Input: part model. Units: mm. Frame: model coordinates. A direction names the side the tool comes from. Round coordinates to 2 decimals unless told otherwise and drop trailing zeros. Order: outer loops, then holes, each group sorted by start corner. A loop starts at its lowest first (then second) coordinate and runs counter-clockwise, first axis right, second up.
Item 1: Cut plane B-B on z = 20.5. Output: boundary loops of the cut face in (x, y).
Item 2: Cut plane D-D on y = -0.8. Give the number of separate pieces and of enclosed holes in the cut face, then the cut area to 3 significant figures.
Item 3: Reachability of faces 1 (the cylindrical face through (23.359, -1.479, -10.926)), 2 (the cylindrical face through (79.533, -1.479, -7.956)), 3 (the cylindrical face through (79.588, -1.479, 7.981)) from +Z, -Z, +X, -X, +Y, -Y: full face, straight path, thin tool, end or side. Return the list, or none.
Item 4: Cut plane A-A on x = 105. Output: boundary loops of the cut face in (y, z).
Item 5: Line query: L1, parallel to X at y = -1.85, z = 22; L2, parallel to X at y = -0.3, z = -17; L3, parallel to X at y = -0.55, z = 5. Output: solid intervals per line, ascending.
Item 6: Cut plane C-C on z = 4. Output: boundary loops of the cut face in (x, y), then the cut area to 3 significant figures.
Item 7: First-contact query: pin 1 (12 mm diameter, centred on x = 19.5, z = 5.5, fed in from +Y); pin 2 (1.5 mm diameter, centred on x = 38, y = -1.5, fed in from -Z); pin 3 (0.9 mm diameter, centred on x = 65, y = -1.5, fed in from +Z); pin 4 (8 mm diameter, centred on x = 105, z = -22, fed in from -Y). Flat tips, straight axial feed; report the tip coordinate or a pass-through.
```python
from build123d import *

# Parameters (mm, degrees)
BASE_DEPTH    = 3
SKETCH2_R     = 6.5
HOLES_DEPTH   = 120.406867474
CUTAWAY_DEPTH = 120.406867474


with BuildPart() as part:
    # Sketch1 → base (new body)
    with BuildSketch(Plane(origin=(0, 0, 0), x_dir=(1, 0, 0), z_dir=(0, 1, 0))):
        with BuildLine():
            Line((-10, -22), (-10, 22))
            ThreePointArc((-10, 22), (-7.071067812, 29.071067812), (0, 32))
            Line((0, 32), (17, 32))
            ThreePointArc((17, 32), (21.226182617, 31.06307787), (24.660444431, 28.427876097))
            Line((24.660444431, 28.427876097), (40.722333621, 9.286061952))
            ThreePointArc((40.722333621, 9.286061952), (42.439464527, 7.968461065), (44.552555836, 7.5))
            Line((44.552555836, 7.5), (77.447444164, 7.5))
            ThreePointArc((77.447444164, 7.5), (79.560535473, 7.968461065), (81.277666379, 9.286061952))
            Line((81.277666379, 9.286061952), (97.339555569, 28.427876097))
            ThreePointArc((97.339555569, 28.427876097), (108.420201433, 31.396926208), (115, 22))
            Line((115, 22), (115, -22))
            ThreePointArc((115, -22), (108.420201433, -31.396926208), (97.339555569, -28.427876097))
            Line((97.339555569, -28.427876097), (81.277666379, -9.286061952))
            ThreePointArc((81.277666379, -9.286061952), (79.560535473, -7.968461065), (77.447444164, -7.5))
            Line((77.447444164, -7.5), (44.552555836, -7.5))
            ThreePointArc((44.552555836, -7.5), (42.439464527, -7.968461065), (40.722333621, -9.286061952))
            Line((40.722333621, -9.286061952), (24.660444431, -28.427876097))
            ThreePointArc((24.660444431, -28.427876097), (21.226182617, -31.06307787), (17, -32))
            Line((17, -32), (0, -32))
            ThreePointArc((0, -32), (-7.071067812, -29.071067812), (-10, -22))
        make_face()
    extrude(amount=-BASE_DEPTH)

    # Sketch2 → holes (cut, through all)
    with BuildSketch(Plane(origin=(0, 0, 0), x_dir=(1, 0, 0), z_dir=(0, 1, 0))):
        with Locations(Location((0, 22, 0), (0, 0, 270))):
            Circle(SKETCH2_R)
        with Locations(Location((17, 22, 0), (0, 0, 270))):
            Circle(SKETCH2_R)
        with Locations(Location((105, 22, 0), (0, 0, 270))):
            Circle(SKETCH2_R)
        with Locations(Location((105, -22, 0), (0, 0, 270))):
            Circle(SKETCH2_R)
        with Locations(Location((17, -22, 0), (0, 0, 270))):
            Circle(SKETCH2_R)
        with Locations(Location((0, -22, 0), (0, 0, 270))):
            Circle(SKETCH2_R)
    extrude(amount=-HOLES_DEPTH, mode=Mode.SUBTRACT)

    # Sketch3 → cutaway (cut, through all)
    with BuildSketch(Plane(origin=(0, 0, 0), x_dir=(-1, 0, 0), z_dir=(0, 1, 0))):
        with BuildLine():
            Line((-21, -7.616814662), (-21, 7.616814662))
            ThreePointArc((-21, 7.616814662), (-23.302929498, 10.905738834), (-27.181155551, 9.866571295))
            Line((-27.181155551, 9.866571295), (-33.572421924, 2.249756634))
            ThreePointArc((-33.572421924, 2.249756634), (-34.391266373, 0), (-33.572421924, -2.249756634))
            Line((-33.572421924, -2.249756634), (-27.181155551, -9.866571295))
            ThreePointArc((-27.181155551, -9.866571295), (-23.302929498, -10.905738834), (-21, -7.616814662))
        make_face()
        with BuildLine():
            Line((-94.818844449, -9.866571295), (-88.427578076, -2.249756634))
            ThreePointArc((-88.427578076, -2.249756634), (-87.608733627, 0), (-88.427578076, 2.249756634))
            Line((-88.427578076, 2.249756634), (-94.818844449, 9.866571295))
            ThreePointArc((-94.818844449, 9.866571295), (-98.697070502, 10.905738834), (-101, 7.616814662))
            Line((-101, 7.616814662), (-101, -7.616814662))
            ThreePointArc((-101, -7.616814662), (-98.697070502, -10.905738834), (-94.818844449, -9.866571295))
        make_face()
    extrude(amount=-CUTAWAY_DEPTH, mode=Mode.SUBTRACT)


solid = part.part
```
From the geometry:
1. outline: (-10, -3) - (-6.32, -3) - (-6.32, 0) - (-10, 0) - close; (6.32, -3) - (10.68, -3) - (10.68, 0) - (6.32, 0) - close; (23.32, -3) - (31.31, -3) - (31.31, 0) - (23.32, 0) - close; (90.69, -3) - (98.68, -3) - (98.68, 0) - (90.69, 0) - close; (111.32, -3) - (115, -3) - (115, 0) - (111.32, 0) - close
2. separate pieces: 1
2. enclosed holes: 8
2. area: 3,840 mm2
3. face 1: +Y, -Y
3. face 2: -Z, +Y, -Y
3. face 3: +Z, +Y, -Y
4. outline: (-3, -32) - (0, -32) - (0, -28.5) - (-3, -28.5) - close; (-3, -15.5) - (0, -15.5) - (0, 15.5) - (-3, 15.5) - close; (-3, 28.5) - (0, 28.5) - (0, 32) - (-3, 32) - close
5. L1: x = -10 to -6.5, 6.5 to 10.5, 23.5 to 30.05, 91.95 to 98.5, 111.5 to 115
5. L2: x = -10 to -4.15, 4.15 to 12.85, 21.15 to 34.25, 87.75 to 100.85, 109.15 to 115
5. L3: x = -10 to 21, 31.26 to 90.74, 101 to 115
6. outline: (-10, -3) - (21, -3) - (21, 0) - (-10, 0) - close; (32.1, -3) - (89.9, -3) - (89.9, 0) - (32.1, 0) - close; (101, -3) - (115, -3) - (115, 0) - (101, 0) - close
6. area: 308 mm2
7. pin 1: stops at y = 0
7. pin 2: stops at z = -13.42
7. pin 3: stops at z = 7.5
7. pin 4: passes through
